Build history of the part. All positions in model axes, mm. Round coordinates to 2 decimals unless told otherwise and drop trailing zeros. Loops run counter-clockwise (first coordinate to the right, second up) from the corner with the lowest first, then second, coordinate; pieces in that order, holes last. Notation, with made-up numbers: (80.25, 7.25) - (113.25, 7.25) arc R17 cw to (113.25, 38.25) - close; hole circle Ø6 at (86, 32). An arc over 180 degrees is marked (long way). Use one line per item in the form item = value. Start each with the question number.
Q1. Saw through at A-A (x = -5). Give the cut face in (y, z).
Q2. Saw through at B-B (x = 8.5). Give the cut face in (y, z).
Q3. Saw through at C-C (z = 1.2). Count the separate pieces of the cut face and the enclosed holes in it, then the cut area to 3 significant figures.
Q4. Pin check, flat tip, straight feed: pin 1 (2.5 mm diameter, centred on x = -38.57, y = 86.55, fed in from +Z). Stop position of the tip, or through.
Q5. Mould opens along Y. For faces 1 (the face through (-31.52, 47.32, 0.99)), 2 (the face through (-17, 38, 2)), 3 (the face through (-26.56, 49.94, 1.01)), 4 (the face through (-39.756, 85.633, 1.014)) say: released by +Y, released by -Y, zero draft, split by the parting line, or undercut.
Q6. Drill centre lines: line 1 (X direction, y = 87, z = 1.4); line 2 (X direction, y = 29, z = 1.2); line 3 (X direction, y = 76.5, z = 0.65). Where is each one in solid material? Low to high.
Autodesk Inventor part; units mm, degrees
ref_plane "YZ Plane" through (0, 0, 0) normal (1, 0, 0) x (0, 1, 0)
ref_plane "XZ Plane" through (0, 0, 0) normal (0, 1, 0) x (-1, 0, 0)
ref_plane "XY Plane" through (0, 0, 0) normal (0, 0, 1) x (1, 0, 0)
sketch "Эскиз1" plane through (0, 0, 0) normal (0, 0, 1) x (1, 0, 0)
  line L0 (15, -22.25) -> (15, 22.25)
  line L1 (15, 22.25) -> (-20, 22.25)
  line L2 (-20, 22.25) -> (-20, -22.25)
  line L3 (-20, -22.25) -> (15, -22.25)
  circle A0 centre (8.763, 2.3275) radius 1.5
  circle A1 centre (8.763, 7.3275) radius 1.5
  circle A2 centre (-11.237, -7.6725) radius 1.5
  circle A3 centre (-11.237, -2.6725) radius 1.5
  circle A4 centre (8.763, -2.6725) radius 1.5
  circle A5 centre (8.763, -7.6725) radius 1.5
  circle A6 centre (-11.237, 2.3275) radius 1.5
  circle A7 centre (-11.237, 7.3275) radius 1.5
  line L4 (-25, 92.25) -> (-62.0049, 92.25)
  line L5 (-103.637, 92.25) -> (-67.893, 92.25)
  circle A8 centre (-49, 104.25) radius 1.5
  circle A9 centre (-42, 104.25) radius 1.5
  circle A10 centre (-35, 104.25) radius 1.5
  circle A11 centre (-35, 111.25) radius 1.5
  circle A12 centre (-42, 118.25) radius 1.5
  circle A13 centre (-49, 118.25) radius 1.5
  circle A14 centre (-49, 111.25) radius 1.5
  circle A15 centre (-35, 118.25) radius 1.5
  circle A16 centre (-42, 111.25) radius 1.5
  circle A17 centre (-42, 97.25) radius 1.5
  circle A18 centre (-35, 97.25) radius 1.5
  circle A19 centre (-49, 97.25) radius 1.5
  line L6 (-25, 92.25) -> (-62.0049, 92.25)
  line L7 (-25, 95.25) -> (-25, 92.25)
  line L8 (-20, 95.25) -> (-25, 95.25)
  line L9 (-20, 95.25) -> (-20, 123.25)
  line L10 (-28, 123.25) -> (-20, 123.25)
  line L11 (-28, 129.25) -> (-28, 123.25)
  line L12 (-28, 129.25) -> (-62.0049, 129.25)
  line L13 (-62.0049, 92.25) -> (-62.0049, 129.25)
  line L14 (-5.1452, 11.625) -> (-40, 100) construction
  arc A20 (-32.5697, 102.9649) -> (-47.4303, 97.0351) centre (-40, 100) ccw
  line L15 (-5.1452, 11.625) -> (-22.5726, 55.8125) construction
  arc A21 (-13.8135, 8.0713) -> (-4.3725, 15.1785) centre (-0.8009, 0.6099) ccw
  line L16 (12.7625, 7.0157) -> (-32.7662, 103.4164)
  line L17 (-47.6184, 97.5588) -> (-15.0854, -3.9674)
  point P0 (0, 0)
  point P1 (-13.8589, 33.7187)
  point P2 (-33.6095, 104.8127)
  point P3 (-34.2206, 105.5316)
  point P4 (-47.7749, 98.1155)
  point P5 (-47.5011, 97.1926)
  dimension "d0" = 8
  dimension "d1" = 95
  dimension "d2" = 100
  dimension "d3" = 40
  dimension "d4" = 15
extrude "Выдавливание1" add sketch "Эскиз1" along normal blind 2 contours L16 A21 L17 L2 L1 | L1 L2 L17 L4 L16 | L4 L17 A19 A20 A10 L16 | A20 A10 | A10 A20 | A1 | A2 | A3 | A4 | A5 | A7 | A9
sketch "Эскиз2" plane through (0, 0, 2) normal (0, 0, 1) x (1, 0, 0)
  circle A0 centre (-38.5661, 86.5462) radius 1.5
  line L0 (-47.5011, 97.1926) -> (-15.0854, -3.9674)
  circle A1 centre (-35.5146, 77.0232) radius 1.5
  circle A2 centre (-32.463, 67.5001) radius 1.5
  circle A3 centre (-29.4114, 57.9771) radius 1.5
  circle A4 centre (-26.3599, 48.4541) radius 1.5
  circle A5 centre (-23.3083, 38.9311) radius 1.5
  circle A6 centre (-20.2568, 29.408) radius 1.5
  circle A7 centre (-17.2052, 19.885) radius 1.5
  circle A8 centre (-42, 97.25) radius 1.5
  circle A9 centre (-11.237, 2.3275) radius 1.5
  point P0 (0, 0)
  dimension "d7" = 3
  dimension "d10" = 10
  dimension "d17" = 5.2562
  dimension "d18" = 5.26
extrude "Выдавливание2" cut sketch "Эскиз2" against normal blind 3 contours A0 | A1 | A2 | A3 | A4 | A5 | A6 | A7
sketch "Эскиз3" plane through (0, 0, 2) normal (0, 0, 1) x (1, 0, 0)
  circle A0 centre (-35, 97.25) radius 1.5
  line L0 (12.7625, 7.0157) -> (-32.7662, 103.4164)
  circle A1 centre (-30.5318, 87.7899) radius 1.5
  circle A2 centre (-26.2613, 78.7476) radius 1.5
  circle A3 centre (-21.9908, 69.7054) radius 1.5
  circle A4 centre (-17.7202, 60.6631) radius 1.5
  circle A5 centre (-13.4497, 51.6208) radius 1.5
  circle A6 centre (-9.1792, 42.5786) radius 1.5
  circle A7 centre (-4.9086, 33.5363) radius 1.5
  circle A8 centre (-0.6381, 24.494) radius 1.5
  point P0 (0, 0)
  dimension "d19" = 3
  dimension "d20" = 4.6533
  dimension "d21" = 4.653
  dimension "d24" = 10
extrude "Выдавливание3" cut sketch "Эскиз3" against normal blind 3 contours A1 | A2 | A3 | A4 | A5 | A6 | A7 | A8
sketch "Эскиз4" plane through (0, 0, 0) normal (0, 0, -1) x (-1, 0, 0)
  circle A0 centre (42, 97.25) radius 1.5
  circle A1 centre (35, 97.25) radius 1.5 construction
  arc A2 (35, 97.25) -> (36.2942, 93.1949) centre (42, 97.25) ccw construction
  arc A3 (33.5, 97.25) -> (35.0715, 92.326) centre (42, 97.25) ccw
  arc A4 (36.5, 97.25) -> (37.5169, 94.0639) centre (42, 97.25) ccw
  arc A5 (36.5, 97.25) -> (33.5, 97.25) centre (35, 97.25) ccw construction
  arc A6 (35.0715, 92.326) -> (37.5169, 94.0639) centre (36.2942, 93.1949) ccw
  arc A7 (36.7604, 101.8918) -> (35.0715, 96.252) centre (42, 97.25) ccw construction
  arc A8 (35.6376, 102.8865) -> (33.5868, 96.0382) centre (42, 97.25) ccw
  arc A9 (37.8832, 100.8971) -> (36.5562, 96.4659) centre (42, 97.25) ccw
  arc A10 (37.8832, 100.8971) -> (35.6376, 102.8865) centre (36.7604, 101.8918) ccw
  arc A11 (33.5868, 96.0382) -> (36.5562, 96.4659) centre (35.0715, 96.252) ccw construction
  point P0 (0, 0)
extrude "Выдавливание4" cut sketch "Эскиз4" against normal blind 3 contours A8 A10 A9 A4 A6 A3
sketch "Эскиз5" plane through (0, 0, 2) normal (0, 0, 1) x (1, 0, 0)
  circle A0 centre (-42, 97.25) radius 1.5
  circle A1 centre (-11.237, 2.3275) radius 1.5
  circle A2 centre (8.763, 2.3275) radius 1.5
  arc A3 (-15.0854, -3.9674) -> (12.7625, 7.0157) centre (-0.8009, 0.6099) ccw
  line L0 (12.7625, 7.0157) -> (-32.7662, 103.4164)
  arc A4 (-32.7662, 103.4164) -> (-33.6095, 104.8127) centre (-40, 100) ccw
  arc A5 (-33.6095, 104.8127) -> (-34.2206, 105.5316) centre (-35, 104.25) ccw
  arc A6 (-34.2206, 105.5316) -> (-47.7749, 98.1155) centre (-40, 100) ccw
  arc A7 (-47.5011, 97.1926) -> (-47.7749, 98.1155) centre (-49, 97.25) ccw
  line L1 (-47.5011, 97.1926) -> (-15.0854, -3.9674)
  circle A8 centre (-17.2052, 19.885) radius 1.5
  circle A9 centre (-23.3083, 38.9311) radius 1.5
  circle A10 centre (-38.5661, 86.5462) radius 1.5
  circle A11 centre (-32.463, 67.5001) radius 1.5
  circle A12 centre (-29.4114, 57.9771) radius 1.5
  circle A13 centre (-35.5146, 77.0232) radius 1.5
  circle A14 centre (-20.2568, 29.408) radius 1.5
  circle A15 centre (-26.3599, 48.4541) radius 1.5
  circle A16 centre (-0.6381, 24.494) radius 1.5
  circle A17 centre (-26.2613, 78.7476) radius 1.5
  circle A18 centre (-4.9086, 33.5363) radius 1.5
  circle A19 centre (-13.4497, 51.6208) radius 1.5
  circle A20 centre (-17.7202, 60.6631) radius 1.5
  circle A21 centre (-9.1792, 42.5786) radius 1.5
  circle A22 centre (-30.5318, 87.7899) radius 1.5
  circle A23 centre (-21.9908, 69.7054) radius 1.5
  circle A24 centre (-23.3083, 38.9311) radius 1.5
  circle A25 centre (-9.1792, 42.5786) radius 1.5
  arc A26 (-9.149, 35.4026) -> (-9.1792, 42.5786) centre (-23.3083, 38.9311) ccw construction
  arc A27 (-7.6935, 35.0399) -> (-7.7268, 42.9535) centre (-23.3083, 38.9311) ccw
  arc A28 (-10.6045, 35.7653) -> (-10.6316, 42.2036) centre (-23.3083, 38.9311) ccw
  arc A29 (-10.6045, 35.7653) -> (-7.6935, 35.0399) centre (-9.149, 35.4026) ccw
  arc A30 (-7.7268, 42.9535) -> (-10.6316, 42.2036) centre (-9.1792, 42.5786) ccw
  arc A31 (-9.1792, 42.5786) -> (-11.0829, 46.8983) centre (-23.3083, 38.9311) ccw construction
  arc A32 (-7.7268, 42.9535) -> (-9.8263, 47.7173) centre (-23.3083, 38.9311) ccw
  arc A33 (-10.6316, 42.2036) -> (-12.3396, 46.0794) centre (-23.3083, 38.9311) ccw
  arc A34 (-10.6316, 42.2036) -> (-7.7268, 42.9535) centre (-9.1792, 42.5786) ccw
  arc A35 (-9.8263, 47.7173) -> (-12.3396, 46.0794) centre (-11.0829, 46.8983) ccw
  point P0 (0, 0)
  point P1 (-10.6316, 42.2036)
  point P2 (-10.6316, 42.2036)
  point P3 (-10.6316, 42.2036)
  point P4 (-7.7268, 42.9535)
  point P5 (-7.7268, 42.9535)
  point P6 (-7.7268, 42.9535)
extrude "Выдавливание5" cut sketch "Эскиз5" against normal blind 3 contours A21 A27 A29 A28 | A21 A33 A35 A32
properties part number "ЛЦМК.30000.30.00.02 Штанга"
Report:
q1.outline = (-13.79, 0) - (32.04, 0) - (32.04, 2) - (-13.79, 2) - close; (35.03, 0) - (44.63, 0) - (44.63, 2) - (35.03, 2) - close
q2.outline = (-11.16, 0) - (0.85, 0) - (0.85, 2) - (-11.16, 2) - close; (3.8, 0) - (16.04, 0) - (16.04, 2) - (3.8, 2) - close
q3.separate_pieces = 1
q3.enclosed_holes = 20
q3.area = 2,710 mm²
q4.pin_1 = through
q5.face_1 = released by -Y
q5.face_2 = zero draft
q5.face_3 = undercut
q5.face_4 = undercut
q6.line_1 = -44.23 to -40, -37.14 to -31.81, -29.26 to -25.01
q6.line_2 = -25.65 to -21.7, -18.81 to 2.38
q6.line_3 = -40.87 to -36.92, -34.11 to -20.05
